from build123d import *

# Parameters (mm, degrees)
SKETCH1_W                            = 91
SKETCH1_H                            = 112
BASE_DEPTH                           = 20
SKETCH2_R                            = 1.4
CASE_ASSEMBLY_HOLES_DEPTH            = 10
SKETCH3_W                            = 83
SKETCH3_H                            = 104
MODULE_CUTOUT_DEPTH                  = 6.6
USB_C_AND_MICRO_USB_SLOTS_DEPTH      = 117.344316578
USB_C_AND_MICRO_USB_SLOTS_DEPTH_BACK = 7
SKETCH4_W                            = 10.5
SKETCH4_H                            = 6
SKETCH4_W_2                          = 10
SKETCH5_W                            = 16.5
SKETCH5_H                            = 10
SKETCH5_W_2                          = 16
SKETCH5_H_2                          = 19
HDMI_AND_USB_SLOTS_DEPTH             = 17.5
SKETCH6_W                            = 17.9
SKETCH6_H                            = 16.2
ETHERNET_SLOT_DEPTH                  = 21
SKETCH7_R                            = 3.6
SKETCH7_W                            = 24
SKETCH7_H                            = 5
TALL_COMPONENTS_CUTOUTS_DEPTH        = 3


with BuildPart() as part:
    # Sketch1 → Base (new body)
    with BuildSketch(Plane(origin=(0, 0, 0), x_dir=(1, 0, 0), z_dir=(0, 1, 0))):
        Rectangle(SKETCH1_W, SKETCH1_H)
    extrude(amount=BASE_DEPTH)

    # Sketch2 → Case Assembly Holes (add)
    # profile 1 of 4: a face of its own
    with BuildSketch(Plane(origin=(0, 0, 0), x_dir=(1, 0, 0), z_dir=(0, 1, 0))):
        with BuildLine():
            Line((-45.5, 56), (-50.5, 56))
            ThreePointArc((-50.5, 56), (-54.5, 52), (-50.5, 48))
            Line((-50.5, 48), (-45.5, 48))
            Line((-45.5, 48), (-45.5, 56))
        make_face()
        with Locations(Location((-50.5, 52, 0), (0, 0, 270))):
            Circle(SKETCH2_R, mode=Mode.SUBTRACT)
    # profile 2 of 4: a face of its own
    with BuildSketch(Plane(origin=(0, 0, 0), x_dir=(1, 0, 0), z_dir=(0, 1, 0))):
        with BuildLine():
            Line((45.5, 48), (50.5, 48))
            ThreePointArc((50.5, 48), (54.5, 52), (50.5, 56))
            Line((50.5, 56), (45.5, 56))
            Line((45.5, 56), (45.5, 48))
        make_face()
        with Locations(Location((50.5, 52, 0), (0, 0, 90))):
            Circle(SKETCH2_R, mode=Mode.SUBTRACT)
    # profile 3 of 4: a face of its own
    with BuildSketch(Plane(origin=(0, 0, 0), x_dir=(1, 0, 0), z_dir=(0, 1, 0))):
        with BuildLine():
            Line((45.5, -56), (50.5, -56))
            ThreePointArc((50.5, -56), (54.5, -52), (50.5, -48))
            Line((50.5, -48), (45.5, -48))
            Line((45.5, -48), (45.5, -56))
        make_face()
        with Locations(Location((50.5, -52, 0), (0, 0, 270))):
            Circle(SKETCH2_R, mode=Mode.SUBTRACT)
    # profile 4 of 4: a face of its own
    with BuildSketch(Plane(origin=(0, 0, 0), x_dir=(1, 0, 0), z_dir=(0, 1, 0))):
        with BuildLine():
            Line((-45.5, -48), (-50.5, -48))
            ThreePointArc((-50.5, -48), (-54.5, -52), (-50.5, -56))
            Line((-50.5, -56), (-45.5, -56))
            Line((-45.5, -56), (-45.5, -48))
        make_face()
        with Locations(Location((-50.5, -52, 0), (0, 0, 90))):
            Circle(SKETCH2_R, mode=Mode.SUBTRACT)
    extrude(amount=CASE_ASSEMBLY_HOLES_DEPTH)

    # Sketch3 → Module Cutout (cut)
    with BuildSketch(Plane.XZ):
        Rectangle(SKETCH3_W, SKETCH3_H)
    extrude(amount=-MODULE_CUTOUT_DEPTH, mode=Mode.SUBTRACT)

    # Sketch4 → USB-C and Micro-USB Slots (cut, two sides: drawn at the far end of the back side and taken through both)
    with BuildSketch(Plane.ZY.offset(45.5).offset(-USB_C_AND_MICRO_USB_SLOTS_DEPTH_BACK)):
        with Locations((-44, 3)):
            Rectangle(SKETCH4_W, SKETCH4_H)
        with Locations((42, 3)):
            Rectangle(SKETCH4_W_2, SKETCH4_H)
    extrude(amount=USB_C_AND_MICRO_USB_SLOTS_DEPTH + USB_C_AND_MICRO_USB_SLOTS_DEPTH_BACK, mode=Mode.SUBTRACT)

    # Sketch5 → HDMI and USB Slots (cut)
    with BuildSketch(Plane.ZY.offset(45.5)):
        with Locations((-26.25, 5)):
            Rectangle(SKETCH5_W, SKETCH5_H)
        with Locations((-7.4, 9.5)):
            Rectangle(SKETCH5_W_2, SKETCH5_H_2)
        with Locations((9.6, 9.5)):
            Rectangle(SKETCH5_W_2, SKETCH5_H_2)
    extrude(amount=-HDMI_AND_USB_SLOTS_DEPTH, mode=Mode.SUBTRACT)

    # Sketch6 → Ethernet Slot (cut)
    with BuildSketch(Plane.ZY.offset(45.5)):
        with Locations((26.55, 8.1)):
            Rectangle(SKETCH6_W, SKETCH6_H)
    extrude(amount=-ETHERNET_SLOT_DEPTH, mode=Mode.SUBTRACT)

    # Sketch7 → Tall Components Cutouts (cut)
    with BuildSketch(Plane.XZ.offset(-6.6)):
        with Locations(Location((-20.05, -12.75, 0), (0, 0, 270))):
            Circle(SKETCH7_R)
        with Locations(Location((-15.25, 32.09, 0), (0, 0, 270))):
            Circle(SKETCH7_R)
        with Locations((6.5, -46.25)):
            Rectangle(SKETCH7_W, SKETCH7_H)
    extrude(amount=-TALL_COMPONENTS_CUTOUTS_DEPTH, mode=Mode.SUBTRACT)


solid = part.part
Input: part model. Units: mm. Frame: model coordinates. A direction names the side the tool comes from. Round coordinates to 2 decimals unless told otherwise and drop trailing zeros. Order: outer loops, then holes, each group sorted by start corner. A loop starts at its lowest first (then second) coordinate and runs counter-clockwise, first axis right, second up. Notation, with made-up numbers: (33.25, -29) - (82.25, -29) arc R26 ccw to (82.25, -1) - close; hole circle Ø9 at (84, 70). An arc over 180 degrees is marked (long way). Answer as a JSON object with one key per item and string values. Group by question number.
(1) Draft query along X for faces 1 (the face through (-41.5, 6.2, -41.4)), 2 (the face through (-28, 13, 9)), 3 (the face through (-43, 3, 47)). Return one class per face: released by +X, released by -X, zero draft, split by the parting line, or undercut.
(2) Reachability of faces 4 (the face through (-23.244, 8.079, -14.411)), 5 (the face through (48, 5, 48)), 6 (the face through (48.9, 10, 51.9)), 7 (the face through (-37, 19, 9)) from +Z, -Z, +X, -X, +Y, -Y: full face, straight path, thin tool, end or side. Return the list, or none.
(3) Cut plane B-B (z = -12). Return loops of the section in (x, y), then the cut area to 3 significant figures.
(4) Pin query (flat end, axial travel): P1, Ø7.5, axis at y = 4.5, z = 43, coming from the +X side; P2, Ø7.5, axis at y = 4.5, z = -16.5, coming from the -X side; P3, Ø6.5, axis at x = 50.5, z = -53.5, coming from the +Y side. Return the tip coordinate at first contact, or that it passes through.
(5) Cut plane A-A (x = 29). Return loops of the section in (y, z), then the cut area to 3 significant figures.
(6) Material intervals for probe 1 along X at (y, z) = (8, -52); probe 2 along X at (y, z) = (7.5, -12.75); probe 3 along Z at (x, y) = (11, 3), sorted ascending. Write a range as from..to.
Here are the results:
{
 "1": {"face 1": "undercut", "face 2": "released by -X", "face 3": "zero draft"},
 "2": {"face 4": "-Y", "face 5": "+X, +Y, -Y", "face 6": "+Z, -Z, +X, +Y", "face 7": "-X, -Y"},
 "3": {"outline": "(-45.5, 19) - (-28, 19) - (-28, 6.6) - (-23.57, 6.6) - (-23.57, 9.6) - (-16.53, 9.6) - (-16.53, 6.6) - (41.5, 6.6) - (41.5, 0) - (45.5, 0) - (45.5, 20) - (-45.5, 20) - close", "area": "1,010 mm^2"},
 "4": {"P1": "stops at x = 45.5", "P2": "stops at x = -45.5", "P3": "stops at y = 10"},
 "5": {"outline": "(0, -56) - (20, -56) - (20, 56) - (0, 56) - (0, 52) - (6.6, 52) - (6.6, -52) - (0, -52) - close", "area": "1,550 mm^2"},
 "6": {"probe 1": "x = -54.5..-51.9, -49.1..49.1, 51.9..54.5", "probe 2": "x = -28..-23.65, -16.45..45.5", "probe 3": "z = -56..-52, 52..56"}
}
